The model under review builds one solid part; all positions refer to its coordinate system, in mm. A direction names the side the tool comes from. Give positions to 0.01 mm unless a question says otherwise; leave off trailing zeros. Loops run counter-clockwise (first coordinate to the right, second up) from the corner with the lowest first, then second, coordinate; pieces in that order, holes last. Notation, with made-up numbers: M 57,2.25 L 82,2.25 A23 cw 82,14.25 Z; hole C 16,79.25 d3. An arc over 180 degrees is marked long. Put each result on its own line as item: value. Start each with the question number.
from build123d import *

# Parameters (mm, degrees)
BOSS_EXTRUDE1_DEPTH     = 100
SKETCH3_R               = 6
BOSS_EXTRUDE2_DEPTH     = 4
BOSS_EXTRUDE3_START     = 4
SKETCH4_R               = 6
BOSS_EXTRUDE3_DEPTH     = 4
CUT_EXTRUDE1_DEPTH      = 130.646635128
CUT_EXTRUDE1_DEPTH_BACK = 130.646635128
SKETCH9_R               = 4.1
CUT_EXTRUDE2_DEPTH      = 134.341666406
CUT_EXTRUDE2_DEPTH_BACK = 134.341666406
SKETCH10_R              = 2.55
SKETCH13_W              = 60
SKETCH13_H              = 31.00370213
CUT_EXTRUDE5_DEPTH      = 24
FILLET1_R               = 3
FILLET2_R               = 5
FILLET3_R               = 4


with BuildPart() as part:
    # Sketch2 → Boss-Extrude1 (new body)
    with BuildSketch(Plane.XY):
        Polygon((0, 0), (0, 23.99629787), (7.5, 38), (7.5, 70), (32.5, 70), (32.5, 38), (40, 23.99629787), (40, 0), (44, 0), (44, 25), (36.5, 39.00370213), (36.5, 74), (3.5, 74), (3.5, 39.00370213), (-4, 25), (-4, 0), align=None)
    extrude(amount=BOSS_EXTRUDE1_DEPTH)

    # Sketch3 → Boss-Extrude2 (add)
    with BuildSketch(Plane.ZY.offset(-32.5)):
        with Locations(Location((84, 46, 0), (0, 0, 90))):
            Circle(SKETCH3_R)
        with Locations(Location((16, 46, 0), (0, 0, 90))):
            Circle(SKETCH3_R)
    extrude(amount=BOSS_EXTRUDE2_DEPTH)

    # Sketch4 → Boss-Extrude3 (add)
    with BuildSketch(Plane(origin=(7.5, 0, 0), x_dir=(0, 0, -1), z_dir=(1, 0, 0)).offset(BOSS_EXTRUDE3_START)):
        with Locations(Location((-16, 46, 0), (0, 0, 90))):
            Circle(SKETCH4_R)
        with Locations(Location((-84, 46, 0), (0, 0, 90))):
            Circle(SKETCH4_R)
    extrude(amount=-BOSS_EXTRUDE3_DEPTH)

    # Sketch9 → Cut-Extrude1 (cut, two sides: drawn at the far end of the back side and taken through both)
    with BuildSketch(Plane(origin=(7.5, 0, 0), x_dir=(0, 0, -1), z_dir=(1, 0, 0)).offset(-CUT_EXTRUDE1_DEPTH_BACK)):
        with Locations((-16, 46)):
            Circle(SKETCH9_R)
        with Locations((-84, 46)):
            Circle(SKETCH9_R)
    extrude(amount=CUT_EXTRUDE1_DEPTH + CUT_EXTRUDE1_DEPTH_BACK, mode=Mode.SUBTRACT)

    # Sketch10 → Cut-Extrude2 (cut, two sides: drawn at the far end of the back side and taken through both)
    with BuildSketch(Plane(origin=(44, 0, 0), x_dir=(0, 0, -1), z_dir=(1, 0, 0)).offset(-CUT_EXTRUDE2_DEPTH_BACK)):
        with Locations(Location((-10, 10, 0), (0, 0, 90))):
            Circle(SKETCH10_R)
        with Locations(Location((-90, 10, 0), (0, 0, 90))):
            Circle(SKETCH10_R)
    extrude(amount=CUT_EXTRUDE2_DEPTH + CUT_EXTRUDE2_DEPTH_BACK, mode=Mode.SUBTRACT)

    # Sketch13 → Cut-Extrude5 (cut)
    with BuildSketch(Plane.ZY.offset(4)):
        with Locations((50, 15.501851065)):
            Rectangle(SKETCH13_W, SKETCH13_H)
    extrude(amount=-CUT_EXTRUDE5_DEPTH, mode=Mode.SUBTRACT)

    # Fillet1
    fillet1_edges = [part.edges().sort_by_distance(p)[0] for p in [
        (1.48419643, 31.00370213, 20),
        (1.48419643, 31.00370213, 80),
    ]]
    fillet(fillet1_edges, radius=FILLET1_R)

    # Fillet2
    fillet2_edges = [part.edges().sort_by_distance(p)[0] for p in [
        (32.5, 70, 50),
        (7.5, 70, 50),
    ]]
    fillet(fillet2_edges, radius=FILLET2_R)

    # Fillet3
    fillet3_edges = [part.edges().sort_by_distance(p)[0] for p in [
        (-4, 25, 10),
        (0, 23.99629787, 10),
        (-4, 25, 90),
        (3.5, 39.00370213, 50),
        (36.5, 39.00370213, 50),
        (44, 25, 50),
        (40, 23.99629787, 50),
        (32.5, 38, 50),
        (7.5, 38, 50),
        (0, 23.99629787, 90),
    ]]
    fillet(fillet3_edges, radius=FILLET3_R)


solid = part.part
(1) Draft analysis for pull direction Z (two halves, no side actions). For faces 6 (the flat face through (28.5, 49, 88)), 7 (the flat face through (1, 31.004, 50)), 8 (the flat face through (7, 45, 0)), state which applies: +Z half, -Z half, draft (parallel to the pull), parting line (faces both ways), or undercut.
(2) Insertion check: pin 1 (10.5 mm diameter, centred on y = 46, z = 84, fed in from -X); pin 2 (3.5 mm diameter, centred on y = 49, z = 16.5, fed in from +X); pin 3 (1.5 mm diameter, centred on y = 38.5, z = 18, fed in from +X); pin 4 (1.5 mm diameter, centred on x = 2.5, y = 17.5, fed in from -Z). Each pin has a flat end and moves straight along its axis. Give the tip position at first contact, or say it passes through.
(3) We need section A-A, the plane y = 10. Write out the cut boundary in (x, z), plus the area to 3 significant figures.
(4) We need section D-D, the plane z = 58. Write out the cut boundary in (x, y), plus the area to 3 significant figures.
(5) We need section C-C, the plane z = 16. State how many separate pieces and enclosed holes the cut face has, plus the area to 3 significant figures.
(6) We need section B-B, the plane y = 36. Write out the cut boundary in (x, z), plus the area to 3 significant figures.
(7) To check wall thickness, follow L1, parallel to Z at x = 43.1, y = 10; L2, parallel to X at y = 62, z = 70.5; L3, parallel to Y at x = 30, z = 84. State the ranges of each line that lie inside material, in increasing order. Write a range as [from, to].
(8) For faces 1 (the flat face through (-2, 0, 90)), 2 (the flat face through (-2, 14, 80)), 3 (the cylindrical face through (-2.03, 11.18, 7.74)), 4 (the cylindrical face through (30.53, 41.58, 79.94)), 5 (the flat face through (20, 70, 49)), list the 3-axis set-ups (+Z, -Z, +X, -X, +Y, -Y) from which the entire face can be reached by the end or side of a thin tool; tool diameter is ignored.
Check sheet entries:
1. face 6: draft
1. face 7: undercut
1. face 8: -Z half
2. pin 1: stops at x = 3.5
2. pin 2: stops at x = 36.5
2. pin 3: stops at x = 37.17
2. pin 4: passes through
3. outline: M -4,0 L 0,0 L 0,7.45 L -4,7.45 Z; M -4,12.55 L 0,12.55 L 0,20 L -4,20 Z; M -4,80 L 0,80 L 0,87.45 L -4,87.45 Z; M -4,92.55 L 0,92.55 L 0,100 L -4,100 Z; M 40,0 L 44,0 L 44,7.45 L 40,7.45 Z; M 40,12.55 L 44,12.55 L 44,87.45 L 40,87.45 Z; M 40,92.55 L 44,92.55 L 44,100 L 40,100 Z
3. area: 478 mm²
4. outline: M -0.78,31 L 3.75,31 L 7.03,37.12 A4 ccw 7.5,39 L 7.5,65 A5 cw 12.5,70 L 27.5,70 A5 cw 32.5,65 L 32.5,39 A4 ccw 32.97,37.12 L 39.53,24.88 A4 cw 40,22.99 L 40,0 L 44,0 L 44,24 A4 ccw 43.53,25.88 L 36.97,38.12 A4 cw 36.5,40.01 L 36.5,74 L 3.5,74 L 3.5,40.01 A4 cw 3.03,38.12 Z
4. area: 590 mm²
5. separate pieces: 3
5. enclosed holes: 0
5. area: 683 mm²
6. outline: M 1.89,0 L 6.43,0 L 6.43,100 L 1.89,100 Z; M 33.57,0 L 38.11,0 L 38.11,100 L 33.57,100 Z
6. area: 908 mm²
7. L1: z = [0, 7.45], [12.55, 87.45], [92.55, 100]
7. L2: x = [3.5, 7.5], [32.5, 36.5]
7. L3: y = [40, 41.9], [50.1, 52], [69.33, 74]
8. face 1: +Z, -Z, +X, -X, -Y
8. face 2: -X, -Y
8. face 3: +X, -X
8. face 4: none
8. face 5: +Z, -Z, -Y
